For this review, take the finished solid that the model builds, in its own axes (mm). A direction names the side the tool comes from. Round coordinates to 2 decimals unless told otherwise and drop trailing zeros. Loops run counter-clockwise (first coordinate to the right, second up) from the corner with the lowest first, then second, coordinate; pieces in that order, holes last. Notation, with made-up numbers: (58.5, 81) -> (90.5, 81) arc R19 cw to (90.5, 110) -> close; hole circle Ø9 at (59.25, 48.25). An arc over 180 degrees is marked (long way). One line per question, with ' | ' between items. Start each with the question number.
1. Consider section B-B (x = -1.5). Write out the cut boundary in (y, z).
2. For pin 1 Ø8.5 at (x, z) = (44.45, 0) entering from -Y; pin 2 Ø4 at (y, z) = (-6.5, 94.5) entering from +X; pin 3 Ø2 at (y, z) = (-11.5, 97.5) entering from +X; pin 4 Ø12 at (y, z) = (-21, 20.5) entering from -X (3 decimals), all flat-tipped, find the tip position at first contact; note any pin that passes through.
3. For faces 1 (the face through (-12.415, -12.522, 91.182)), 2 (the face through (13.377, -12.522, 38.607)), list the 3-axis set-ups (+Z, -Z, +X, -X, +Y, -Y) from which the entire face can be reached by the end or side of a thin tool; tool diameter is ignored.
4. Consider section C-C (x = 39). Write out the cut boundary in (y, z).
5. Draft analysis for pull direction X (two halves, no side actions). For faces 3 (the face through (-12.585, -12.522, 30.601)), 4 (the face through (13.26, -12.52, 11.5)), 5 (the face through (41.52, -12.52, -1.22)), state which applies: pulls with the +X half, pulls with the -X half, needs draft (parallel to the pull), parting line crosses it, or undercut.
6. Wall thickness on line 1 along X through (y, z) = (-18.25, 114.3) (3 decimals); line 2 along X through (y, z) = (-16.5, 101); line 3 along Z through (x, y) = (36.5, -11.5): over which ranges is each line inside the solid? List them lowest first.
7. Consider section A-A (y = -14.75). Count the separate pieces of the cut face and the enclosed holes in it, and give its area (3 significant figures).
8. Consider section D-D (z = 40). Write out the cut boundary in (x, y) (3 decimals), and give its area (3 significant figures).
```python
from build123d import *

# Parameters (mm, degrees)
F1_DEPTH = 25.4


with BuildPart() as f1:
    # F0 (on Front) → F1 (new body)
    with BuildSketch(Plane.XZ):
        with BuildLine():
            ThreePointArc((15.874389109, 63.6392674313), (15.7517676472, 65.4741937567), (15.4177611541, 67.2826268644))
            Line((15.4177611541, 67.2826268644), (15.874389109, 63.6392674313))
        make_face()
        with BuildLine():
            Line((-15.875, 63.5), (-15.3865384615, 67.4076923077))
            ThreePointArc((-15.3865384615, 67.4076923077), (-15.7524112928, 65.4690514116), (-15.875, 63.5))
        make_face()
        with BuildLine():
            Line((-15.5606435644, 60.3564356436), (-15.875, 63.5))
            ThreePointArc((-15.875, 63.5), (-15.7962153946, 61.9203784605), (-15.5606435644, 60.3564356436))
        make_face()
        with BuildLine():
            ThreePointArc((15.875, 63.5), (15.8748472765, 63.5696343856), (15.874389109, 63.6392674313))
            Line((15.874389109, 63.6392674313), (15.5339492009, 60.2270735993))
            ThreePointArc((15.5339492009, 60.2270735993), (15.7895070943, 61.8546761054), (15.875, 63.5))
        make_face()
        with BuildLine():
            Line((0.6794904459, -9.5007324841), (0, -9.525))
            ThreePointArc((0, -9.525), (0.3399618281, -9.5189311877), (0.6794904459, -9.5007324841))
        make_face()
        with BuildLine():
            ThreePointArc((0, 104.775), (6.7351920908, 107.5648079092), (9.525, 114.3))
            ThreePointArc((9.525, 114.3), (0, 123.825), (-9.525, 114.3))
            ThreePointArc((-9.525, 114.3), (-6.7351920908, 107.5648079092), (0, 104.775))
        make_face()
        with BuildLine():
            ThreePointArc((3.175, 114.3), (2.2450640303, 112.0549359697), (0, 111.125))
            ThreePointArc((0, 111.125), (-2.2450640303, 116.5450640303), (3.175, 114.3))
        make_face(mode=Mode.SUBTRACT)
        with BuildLine():
            ThreePointArc((0, 47.625), (-10.0526499203, 51.2134278751), (-15.5606435644, 60.3564356436))
            Line((-15.5606435644, 60.3564356436), (-9.525, 0))
            ThreePointArc((-9.525, 0), (-6.7351920908, 6.7351920908), (0, 9.525))
            Line((0, 9.525), (0, 47.625))
        make_face()
        with BuildLine():
            Line((36.5125, 0), (9.525, 0))
            ThreePointArc((9.525, 0), (6.9712901065, -6.4905114784), (0.6794904459, -9.5007324841))
            Line((0.6794904459, -9.5007324841), (44.45, -7.9375))
            ThreePointArc((44.45, -7.9375), (38.8373399243, -5.6126600757), (36.5125, 0))
        make_face()
        with BuildLine():
            ThreePointArc((52.3875, 0), (50.0626600757, 5.6126600757), (44.45, 7.9375))
            ThreePointArc((44.45, 7.9375), (38.8373399243, 5.6126600757), (36.5125, 0))
            ThreePointArc((36.5125, 0), (38.8373399243, -5.6126600757), (44.45, -7.9375))
            ThreePointArc((44.45, -7.9375), (50.0626600757, -5.6126600757), (52.3875, 0))
        make_face()
        with BuildLine():
            ThreePointArc((47.625, 0), (44.45, -3.175), (41.275, 0))
            ThreePointArc((41.275, 0), (44.45, 3.175), (47.625, 0))
        make_face(mode=Mode.SUBTRACT)
        with BuildLine():
            Line((15.4177611541, 67.2826268644), (9.525, 114.3))
            ThreePointArc((9.525, 114.3), (6.7351920908, 107.5648079092), (0, 104.775))
            Line((0, 104.775), (0, 102.8163525843))
            ThreePointArc((0, 102.8163525843), (1.1626238989, 101.6541683696), (1.5881934232, 100.0663216958))
            ThreePointArc((1.5881934232, 100.0663216958), (1.1626238989, 98.478475022), (0, 97.3162908073))
            Line((0, 97.3162908073), (0, 79.375))
            ThreePointArc((0, 79.375), (9.7971022126, 75.9912934973), (15.4177611541, 67.2826268644))
        make_face()
        with BuildLine():
            Line((11.2794016117, 17.5841850976), (15.5339492009, 60.2270735993))
            ThreePointArc((15.5339492009, 60.2270735993), (10.0014478549, 51.1717127789), (0, 47.625))
            Line((0, 47.625), (0, 9.525))
            ThreePointArc((0, 9.525), (6.7351920908, 6.7351920908), (9.525, 0))
            Line((9.525, 0), (36.5125, 0))
            ThreePointArc((36.5125, 0), (38.8373399243, 5.6126600757), (44.45, 7.9375))
            Line((44.45, 7.9375), (18.9065701995, 8.84976535))
            ThreePointArc((18.9065701995, 8.84976535), (13.2019437733, 11.565658071), (11.2794016117, 17.5841850976))
        make_face()
        with BuildLine():
            ThreePointArc((0, 9.525), (-6.7351920908, 6.7351920908), (-9.525, 0))
            ThreePointArc((-9.525, 0), (-6.7351920908, -6.7351920908), (0, -9.525))
            Line((0, -9.525), (0.6794904459, -9.5007324841))
            ThreePointArc((0.6794904459, -9.5007324841), (6.9712901065, -6.4905114784), (9.525, 0))
            Line((9.525, 0), (3.175, 0))
            ThreePointArc((3.175, 0), (-2.2450640303, -2.2450640303), (0, 3.175))
            Line((0, 3.175), (0, 9.525))
        make_face()
        with BuildLine():
            Line((15.874389109, 63.6392674313), (15.4177611541, 67.2826268644))
            ThreePointArc((15.4177611541, 67.2826268644), (9.7971022126, 75.9912934973), (0, 79.375))
            Line((0, 79.375), (0, 66.675))
            ThreePointArc((0, 66.675), (2.2450640303, 65.7450640303), (3.175, 63.5))
            ThreePointArc((3.175, 63.5), (2.2450640303, 61.2549359697), (0, 60.325))
            Line((0, 60.325), (0, 47.625))
            ThreePointArc((0, 47.625), (10.0014478549, 51.1717127789), (15.5339492009, 60.2270735993))
            Line((15.5339492009, 60.2270735993), (15.874389109, 63.6392674313))
        make_face()
        with BuildLine():
            ThreePointArc((0, 79.375), (-9.7463072395, 76.0309664508), (-15.3865384615, 67.4076923077))
            Line((-15.3865384615, 67.4076923077), (-15.875, 63.5))
            Line((-15.875, 63.5), (-15.5606435644, 60.3564356436))
            ThreePointArc((-15.5606435644, 60.3564356436), (-10.0526499203, 51.2134278751), (0, 47.625))
            Line((0, 47.625), (0, 60.325))
            ThreePointArc((0, 60.325), (-3.175, 63.5), (0, 66.675))
            Line((0, 66.675), (0, 79.375))
        make_face()
        with BuildLine():
            ThreePointArc((0, 104.775), (-6.7351920908, 107.5648079092), (-9.525, 114.3))
            Line((-9.525, 114.3), (-15.3865384615, 67.4076923077))
            ThreePointArc((-15.3865384615, 67.4076923077), (-9.7463072395, 76.0309664508), (0, 79.375))
            Line((0, 79.375), (0, 97.3162908073))
            ThreePointArc((0, 97.3162908073), (-4.7618065768, 100.0663216958), (0, 102.8163525843))
            Line((0, 102.8163525843), (0, 104.775))
        make_face()
        with BuildLine():
            ThreePointArc((9.525, 0), (6.7351920908, 6.7351920908), (0, 9.525))
            Line((0, 9.525), (0, 3.175))
            ThreePointArc((0, 3.175), (2.2450640303, 2.2450640303), (3.175, 0))
            Line((3.175, 0), (9.525, 0))
        make_face()
    extrude(amount=F1_DEPTH)


solid = f1.part
```
Answer block:
1) outline: (-25.4, -9.41) -> (0, -9.41) -> (0, -2.8) -> (-25.4, -2.8) -> close; (-25.4, 2.8) -> (0, 2.8) -> (0, 60.7) -> (-25.4, 60.7) -> close; (-25.4, 66.3) -> (0, 66.3) -> (0, 96.89) -> (-25.4, 96.89) -> close; (-25.4, 103.24) -> (0, 103.24) -> (0, 111.5) -> (-25.4, 111.5) -> close; (-25.4, 117.1) -> (0, 117.1) -> (0, 123.71) -> (-25.4, 123.71) -> close
2) pin 1: stops at y = -25.4 | pin 2: stops at x = 12.26 | pin 3: stops at x = 11.76 | pin 4: stops at x = -12.175
3) face 1: +Z, -X, +Y, -Y | face 2: +X, +Y, -Y
4) outline: (-25.4, -8.13) -> (0, -8.13) -> (0, 8.13) -> (-25.4, 8.13) -> close
5) face 3: pulls with the -X half | face 4: pulls with the +X half | face 5: undercut
6) line 1: x = -9.525 to -3.175, 3.175 to 9.525 | line 2: x = -11.19 to -4.62, 1.45 to 11.19 | line 3: z = -8.22 to 8.22
7) separate pieces: 1 | enclosed holes: 5 | area: 3,760 mm2
8) outline: (-13.525, -25.4) -> (13.516, -25.4) -> (13.516, 0) -> (-13.525, 0) -> close | area: 687 mm2
